from build123d import *

# Parameters (mm, degrees)
SKETCH_1_W          = 47
SKETCH_1_H          = 38
EXTRUDE_1_DEPTH     = 15
SKETCH_2_R          = 11
EXTRUDE_2_DEPTH     = 7.7
FILLET_1_R          = 1
SKETCH_3_R          = 1.5
SKETCH_3_W          = 9
SKETCH_3_H          = 6
CUT_EXTRUDE_1_DEPTH = 5
SKETCH_4_W          = 6
SKETCH_4_H          = 4
EXTRUDE_3_DEPTH     = 5
SKETCH_5_R          = 10
CUT_EXTRUDE_2_DEPTH = 1


with BuildPart() as part:
    # 草图1 → 凸台-拉伸1 (new body)
    with BuildSketch(Plane(origin=(0, 0, 0), x_dir=(1, 0, 0), z_dir=(0, 1, 0))):
        Rectangle(SKETCH_1_W, SKETCH_1_H)
    extrude(amount=EXTRUDE_1_DEPTH)

    # 草图2 → 凸台-拉伸2 (add)
    with BuildSketch(Plane(origin=(0, 15, 0), x_dir=(1, 0, 0), z_dir=(0, 1, 0))):
        with Locations(Location((0, 0, 0), (0, 0, 90))):
            Circle(SKETCH_2_R)
    extrude(amount=EXTRUDE_2_DEPTH)

    # 圆角1
    fillet_1_edges = [part.edges().sort_by_distance(p)[0] for p in [
        (-23.5, 15, 0),
        (0, 15, 11),
        (0, 15, 19),
        (23.5, 15, 0),
        (0, 0, 19),
        (-23.5, 0, 0),
        (0, 0, -19),
        (23.5, 0, 0),
        (0, 15, -19),
    ]]
    fillet(fillet_1_edges, radius=FILLET_1_R)

    # 草图3 → 切除-拉伸1 (cut)
    with BuildSketch(Plane.XZ):
        with Locations(Location((19.5, 14, 0), (0, 0, 270))):
            Circle(SKETCH_3_R)
        with Locations(Location((-19.5, 14, 0), (0, 0, 270))):
            Circle(SKETCH_3_R)
        with Locations(Location((-19.5, -14, 0), (0, 0, 270))):
            Circle(SKETCH_3_R)
        with Locations(Location((19.5, -14, 0), (0, 0, 270))):
            Circle(SKETCH_3_R)
        with Locations((-7, 13)):
            Rectangle(SKETCH_3_W, SKETCH_3_H)
    extrude(amount=-CUT_EXTRUDE_1_DEPTH, mode=Mode.SUBTRACT)

    # 草图4 → 凸台-拉伸3 (add)
    with BuildSketch(Plane.XZ.offset(-5)):
        with Locations((-7, 13)):
            Rectangle(SKETCH_4_W, SKETCH_4_H)
    extrude(amount=EXTRUDE_3_DEPTH)

    # 草图5 → 切除-拉伸2 (cut)
    with BuildSketch(Plane(origin=(0, 22.7, 0), x_dir=(1, 0, 0), z_dir=(0, 1, 0))):
        with Locations(Location((0, 0, 0), (0, 0, 270))):
            Circle(SKETCH_5_R)
    extrude(amount=-CUT_EXTRUDE_2_DEPTH, mode=Mode.SUBTRACT)


solid = part.part
Geometry check sheet. Reference: the model listing, model coordinates, mm. A direction names the side the tool comes from. Coordinates: 2 decimals unless noted, no trailing zeros. Order: outer loops, then holes, each group sorted by start corner. A loop starts at its lowest first (then second) coordinate and runs counter-clockwise, first axis right, second up. Notation, with made-up numbers: (44.5, 23.5) - (60.5, 23.5) arc R21 cw to (60.5, 51.5) - close; hole circle Ø9 at (39.25, 28.5). An arc over 180 degrees is marked (long way). Answer in a Markdown table with one row per item. Add a question column.
1) Gauge pin test, flat ends, axial feed: P1, Ø1.5, axis at y = 17.5, z = -10, coming from the +X side; P2, Ø8, axis at x = -18.5, z = 9.5, coming from the +Y side; P3, Ø0.9, axis at x = -20, z = 14, coming from the -Y side. Record the tip position at first contact, or that the pin passes through.
2) Release check for a two-part mould opening along Z. For faces 4 (the cylindrical face through (0.329, 0.301, -18.715)), 5 (the flat face through (0, 0, 0)), 6 (the flat face through (-7.1, 5, 15.7)) record: +Z half, -Z half, draft (parallel to the pull), parting line (faces both ways), or undercut.
3) Cross-section at C-C, the plane z = 14. Record the cut outline in (x, y).
4) Material ranges on line 1 along X through (y, z) = (3.9, -14); line 2 along X through (y, z) = (2.7, 14); line 3 along X through (y, z) = (22, 0), recorded low to high. Write a range as [from, to].
5) Cross-section at A-A, the plane y = 2.5. Record the cut outline in (x, z).
6) Cross-section at D-D, the plane z = 0. Record the cut outline in (x, y).
7) Set-up check for faces 1 (the flat face through (0, 21.7, 0)), 2 (the flat face through (20, 5, -14)), 3 (the flat face through (23.5, 7, 0)): record each of +Z, -Z, +X, -X, +Y, -Y from which the full face is reachable in a straight line by a thin tool's end or side.
8) Cross-section at B-B, the plane x = -14.5. Record the cut outline in (y, z).
Check result:
| question | item | result |
|---|---|---|
| 1 | P1 | stops at x = 5.95 |
| 1 | P2 | stops at y = 15 |
| 1 | P3 | stops at y = 5 |
| 2 | face 4 | -Z half |
| 2 | face 5 | draft |
| 2 | face 6 | undercut |
| 3 | outline | (-23.5, 1) arc R1 ccw to (-22.5, 0) - (-21, 0) - (-21, 5) - (-18, 5) - (-18, 0) - (-11.5, 0) - (-11.5, 5) - (-10, 5) - (-10, 0) - (-4, 0) - (-4, 5) - (-2.5, 5) - (-2.5, 0) - (18, 0) - (18, 5) - (21, 5) - (21, 0) - (22.5, 0) arc R1 ccw to (23.5, 1) - (23.5, 14) arc R1 ccw to (22.5, 15) - (-22.5, 15) arc R1 ccw to (-23.5, 14) - close |
| 4 | line 1 | x = [-23.5, -21], [-18, 18], [21, 23.5] |
| 4 | line 2 | x = [-23.5, -21], [-18, -11.5], [-10, -4], [-2.5, 18], [21, 23.5] |
| 4 | line 3 | x = [-11, -10], [10, 11] |
| 5 | outline | (-23.5, -19) - (23.5, -19) - (23.5, 19) - (-23.5, 19) - close; (-10, 11) - (-4, 11) - (-4, 15) - (-10, 15) - close; hole circle Ø3 at (-19.5, -14); hole circle Ø3 at (-19.5, 14); hole (-11.5, 10) - (-2.5, 10) - (-2.5, 16) - (-11.5, 16) - close; hole circle Ø3 at (19.5, -14); hole circle Ø3 at (19.5, 14) |
| 6 | outline | (-23.5, 1) arc R1 ccw to (-22.5, 0) - (22.5, 0) arc R1 ccw to (23.5, 1) - (23.5, 14) arc R1 ccw to (22.5, 15) - (12, 15) arc R1 cw to (11, 16) - (11, 22.7) - (10, 22.7) - (10, 21.7) - (-10, 21.7) - (-10, 22.7) - (-11, 22.7) - (-11, 16) arc R1 cw to (-12, 15) - (-22.5, 15) arc R1 ccw to (-23.5, 14) - close |
| 7 | face 1 | +Y |
| 7 | face 2 | -Y |
| 7 | face 3 | +Z, -Z, +X, +Y, -Y |
| 8 | outline | (0, -18) arc R1 ccw to (1, -19) - (14, -19) arc R1 ccw to (15, -18) - (15, 18) arc R1 ccw to (14, 19) - (1, 19) arc R1 ccw to (0, 18) - close |
